Input: dimensioned drawing with shaded views. Units: mm. Origin: part minimum x, y, z. Give positions to 0.01 mm unless a question says otherwise; leave off trailing zeros. Loops run counter-clockwise (first coordinate to the right, second up) from the corner with the lowest first, then second, coordinate; pieces in that order, holes last.
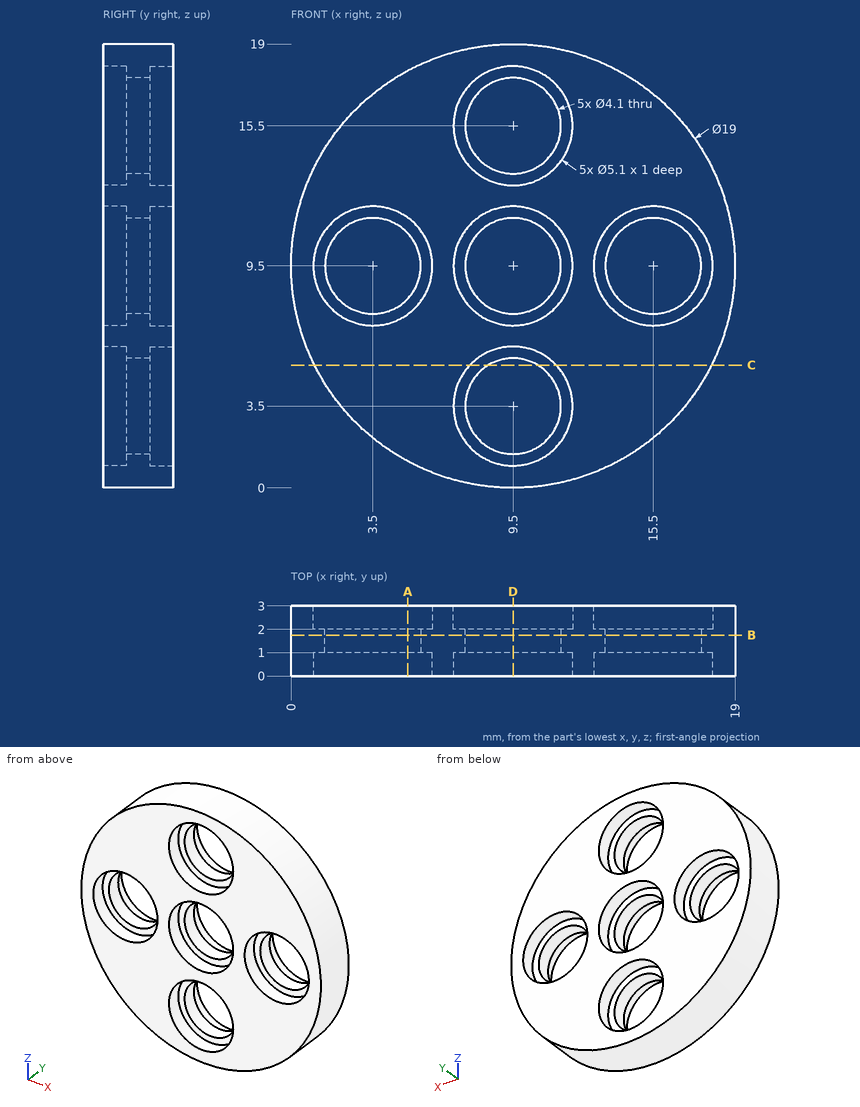
(1) Ray query, line 1 along Z through (x, y) = (9.5, 0.7); line 2 along X through (y, z) = (1.7, 8.25); line 3 along Z through (x, y) = (10, 1.9). Return the intervals inside material, ascending.
A:
line 1: z = 0 to 0.95, 6.05 to 6.95, 12.05 to 12.95, 18.05 to 19
line 2: x = 0.08 to 1.88, 5.12 to 7.88, 11.12 to 13.88, 17.12 to 18.92
line 3: z = 0.01 to 1.51, 5.49 to 7.51, 11.49 to 13.51, 17.49 to 18.99
(2) Section B-B, the plane y = 1.75. Return the cut outline in (x, z), then the cut area to 3 significant figures.
A:
outline: circle Ø19 at (9.5, 9.5); hole circle Ø4.1 at (3.5, 9.5); hole circle Ø4.1 at (9.5, 3.5); hole circle Ø4.1 at (9.5, 9.5); hole circle Ø4.1 at (9.5, 15.5); hole circle Ø4.1 at (15.5, 9.5)
area: 218 mm2
(3) First-contact query: pin 1 (4.5 mm diameter, centred on x = 9.5, z = 3.5, fed in from -Y); pin 2 (4 mm diameter, centred on x = 16, z = 9.5, fed in from +Y); pin 3 (6 mm diameter, centred on x = 9.5, z = 15.5, fed in from +Y); pin 4 (1 mm diameter, centred on y = 0.5, z = 17, fed in from +X). Flat tips, straight axial feed; report the tip coordinate or a pass-through.
A:
pin 1: stops at y = 1
pin 2: stops at y = 2
pin 3: stops at y = 3
pin 4: stops at x = 15.92
(4) Section D-D, the plane x = 9.5. Count the separate pieces of the cut face and the enclosed holes in it, then the cut area to 3 significant figures.
A:
separate pieces: 4
enclosed holes: 0
area: 14.1 mm2
(5) Section C-C, the plane z = 5.25. Return the cut outline in (x, y).
A:
outline: (1, 0) - (7.65, 0) - (7.65, 1) - (8.43, 1) - (8.43, 2) - (7.65, 2) - (7.65, 3) - (1, 3) - close; (10.57, 1) - (11.35, 1) - (11.35, 0) - (18, 0) - (18, 3) - (11.35, 3) - (11.35, 2) - (10.57, 2) - close
(6) Section A-A, the plane x = 5. Return the cut outline in (y, z), then the cut area to 3 significant figures.
A:
outline: (0, 1.13) - (3, 1.13) - (3, 7.44) - (2, 7.44) - (2, 8.1) - (1, 8.1) - (1, 7.44) - (0, 7.44) - close; (0, 11.56) - (1, 11.56) - (1, 10.9) - (2, 10.9) - (2, 11.56) - (3, 11.56) - (3, 17.87) - (0, 17.87) - close
area: 39.2 mm2
